Source: CAD feature listing. Evaluate the final solid. Frame: model axes, mm. Face numbers are marked on the shaded views. A direction names the side the tool comes from. Round coordinates to 2 decimals unless told otherwise and drop trailing zeros. Write each loop counter-clockwise with the first axis right and the second up, starting at its lowest first coordinate (ties: lowest second). Pieces come first, ordered by that corner, then holes. Notation, with made-up numbers: (51, 10) -> (62, 10) arc R19 ccw to (62, 25) -> close; hole circle Ø6 at (65, 40.25). An arc over 180 degrees is marked (long way). Return JSON: item names as keys, results as strings. Group by question number.
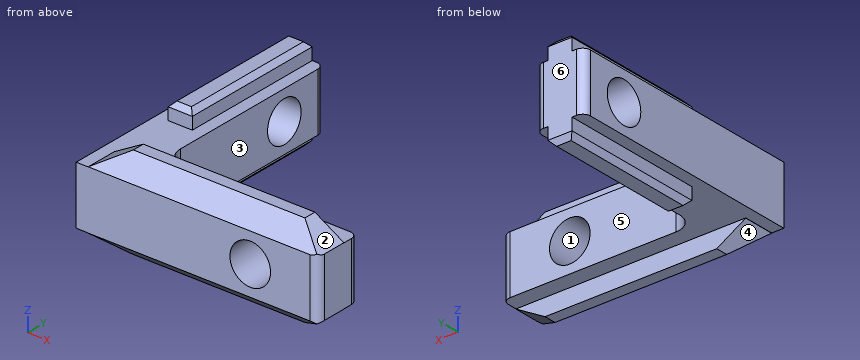
from build123d import *

# Parameters (mm, degrees)
EXTRUDE1_DEPTH        = 3
EXTRUDE1_DEPTH_BACK   = 3
SKETCH2_W             = 2.5
SKETCH2_H             = 15
SKETCH2_W_2           = 23.75
SKETCH2_H_2           = 3.25
EXTRUDE2_DEPTH        = 1.75
CHAMFER1_SIZE         = 3
CHAMFER1_SIZE2        = 1.732050808
CHAMFER2_SIZE         = 2
CHAMFER2_SIZE2        = 1.738573476
CHAMFER3_SIZE         = 0.5
FILLET1_R             = 0.8
FILETE1_R             = 2
FURO_ROSCADO_DE_M51_D = 4.2
FURO_ROSCADO_DE_M52_D = 4.2


# Read off the part's stored shape, not the designer's step: Mirror1
with BuildPart() as part:
    # Sketch1 → Extrude1 (new, two sides: drawn at the far end of the back side and taken through both)
    with BuildSketch(Plane.XY.offset(-EXTRUDE1_DEPTH_BACK)):
        Polygon((0, 0), (0, 20), (-5, 20), (-5, -5), (20, -5), (20, 0), align=None)
    extrude(amount=EXTRUDE1_DEPTH + EXTRUDE1_DEPTH_BACK)

    # Sketch2 → Extrude2 (add)
    with BuildSketch(Plane.XY.offset(3)):
        with Locations((-2.5, 12.5)):
            Rectangle(SKETCH2_W, SKETCH2_H)
        with Locations((8.125, -3.375)):
            Rectangle(SKETCH2_W_2, SKETCH2_H_2)
    extrude(amount=EXTRUDE2_DEPTH)

    # Chamfer1
    chamfer1_edges = [part.edges().sort_by_distance(p)[0] for p in [
        (20, -3.375, 4.75),
        (-3.75, -3.375, 4.75),
    ]]
    chamfer1_side = [part.faces().sort_by_distance(p)[0] for p in [
        (8.125, -3.375, 4.75),
    ]]
    chamfer(chamfer1_edges, length=CHAMFER1_SIZE, length2=CHAMFER1_SIZE2, reference=chamfer1_side[0])

    # Chamfer2
    chamfer2_edges = [part.edges().sort_by_distance(p)[0] for p in [
        (8.125, -5, 4.75),
    ]]
    chamfer2_side = [part.faces().sort_by_distance(p)[0] for p in [
        (8.125, -3.375, 4.75),
    ]]
    chamfer(chamfer2_edges, length=CHAMFER2_SIZE, length2=CHAMFER2_SIZE2, reference=chamfer2_side[0])

    # Chamfer3
    chamfer3_edges = [part.edges().sort_by_distance(p)[0] for p in [
        (-2.5, 20, 4.75),
        (-1.25, 12.5, 4.75),
        (-2.5, 5, 4.75),
        (-3.75, 12.5, 4.75),
    ]]
    chamfer(chamfer3_edges, length=CHAMFER3_SIZE)

    # Mirror1: part across plane


with BuildPart() as part_1:
    add(part.part)
    add(part.part.mirror(Plane.XY))

    # Fillet1
    fillet1_edges = [part_1.edges().sort_by_distance(p)[0] for p in [
        (-5, 20, 0),
        (20, -5, 0),
        (20, 0, 0),
        (0, 20, 0),
    ]]
    fillet(fillet1_edges, radius=FILLET1_R)

    # Filete1
    filete1_edges = [part_1.edges().sort_by_distance(p)[0] for p in [
        (0, 0, 0),
    ]]
    fillet(filete1_edges, radius=FILETE1_R)

    # Furo roscado de M51 (through all)
    with Locations(Plane(origin=(0, 0, 0), x_dir=(1, 0, 0), z_dir=(0, 1, 0))):
        with Locations((13, 0)):
            Hole(FURO_ROSCADO_DE_M51_D / 2)

    # Furo roscado de M52 (through all)
    with Locations(Plane(origin=(0, 0, 0), x_dir=(0, 0, -1), z_dir=(1, 0, 0))):
        with Locations((0, 15)):
            Hole(FURO_ROSCADO_DE_M52_D / 2)


solid = part_1.part
Item 1: Pull-direction query (Z, two-part tool) for the marked faces 1, 2, 3 and 4; classes: +Z half, -Z half, draft (parallel to the pull), parting line (faces both ways), or undercut.
Item 2: Cut plane B-B on y = 15. Output: boundary loops of the cut face in (x, z), and give its area (4 significant figures).
Item 3: Material intervals for probe 1 along Y at (x, z) = (-3.2, 0); probe 2 along Z at (x, y) = (13, -2.4); probe 3 along X at (y, z) = (17, -2.75), sorted ascending.
Item 4: Set-up query: the marked faces 5 and 6. Return all of +Z, -Z, +X, -X, +Y, -Y with unobstructed straight access to the full face (end or side cutting, diameter ignored); none if empty.
Item 5: Cut plane D-D on z = 3.5. Output: boundary loops of the cut face in (x, y).
Item 6: First-contact query: pin 1 Ø4 at (y, z) = (7.5, 2) entering from +X; pin 2 Ø0.9 at (x, z) = (10.5, -3.5) entering from +Y; pin 3 Ø4 at (y, z) = (15, 0) entering from -X; pin 4 Ø1.8 at (x, z) = (14, -1.5) entering from +Y. Flat tips, straight axial feed; report the tip coordinate or a pass-through.
Item 7: Cut plane A-A on x = 13. Output: boundary loops of the cut face in (y, z).
Item 8: Cut plane C-C on z = 0. Output: boundary loops of the cut face in (x, y), and give its area (3 significant figures).
Here are the results:
{
 "1": {"face 1": "undercut", "face 2": "+Z half", "face 3": "draft", "face 4": "-Z half"},
 "2": {"outline": "(-5, -3) -> (-3.75, -3) -> (-3.75, -4.25) -> (-3.25, -4.75) -> (-1.75, -4.75) -> (-1.25, -4.25) -> (-1.25, -3) -> (0, -3) -> (0, -2.1) -> (-5, -2.1) -> close; (-5, 2.1) -> (0, 2.1) -> (0, 3) -> (-1.25, 3) -> (-1.25, 4.25) -> (-1.75, 4.75) -> (-3.25, 4.75) -> (-3.75, 4.25) -> (-3.75, 3) -> (-5, 3) -> close", "area": "17.25 mm^2"},
 "3": {"probe 1": "y = -5 to 12.9, 17.1 to 20", "probe 2": "z = -4.75 to -2.1, 2.1 to 4.75", "probe 3": "x = -5 to 0"},
 "4": {"face 5": "+Z, -Z, +X, +Y", "face 6": "+Z, -Z, +X, -X, +Y"},
 "5": {"outline": "(-3.75, 5) -> (-1.25, 5) -> (-1.25, 20) -> (-3.75, 20) -> close; (-2.92, -4.44) -> (19.17, -4.44) -> (19.17, -1.75) -> (-2.92, -1.75) -> close"},
 "6": {"pin 1": "stops at x = 0", "pin 2": "stops at y = -1.75", "pin 3": "passes through", "pin 4": "stops at y = 0"},
 "7": {"outline": "(-5, -3.01) -> (-3, -4.75) -> (-1.75, -4.75) -> (-1.75, -3) -> (0, -3) -> (0, -2.1) -> (-5, -2.1) -> close; (-5, 2.1) -> (0, 2.1) -> (0, 3) -> (-1.75, 3) -> (-1.75, 4.75) -> (-3, 4.75) -> (-5, 3.01) -> close"},
 "8": {"outline": "(-5, -5) -> (10.9, -5) -> (10.9, 0) -> (2, 0) arc R2 cw to (0, 2) -> (0, 12.9) -> (-5, 12.9) -> close; (-5, 17.1) -> (0, 17.1) -> (0, 19.2) arc R0.8 ccw to (-0.8, 20) -> (-4.2, 20) arc R0.8 ccw to (-5, 19.2) -> close; (15.1, -5) -> (19.2, -5) arc R0.8 ccw to (20, -4.2) -> (20, -0.8) arc R0.8 ccw to (19.2, 0) -> (15.1, 0) -> close", "area": "183 mm^2"}
}
